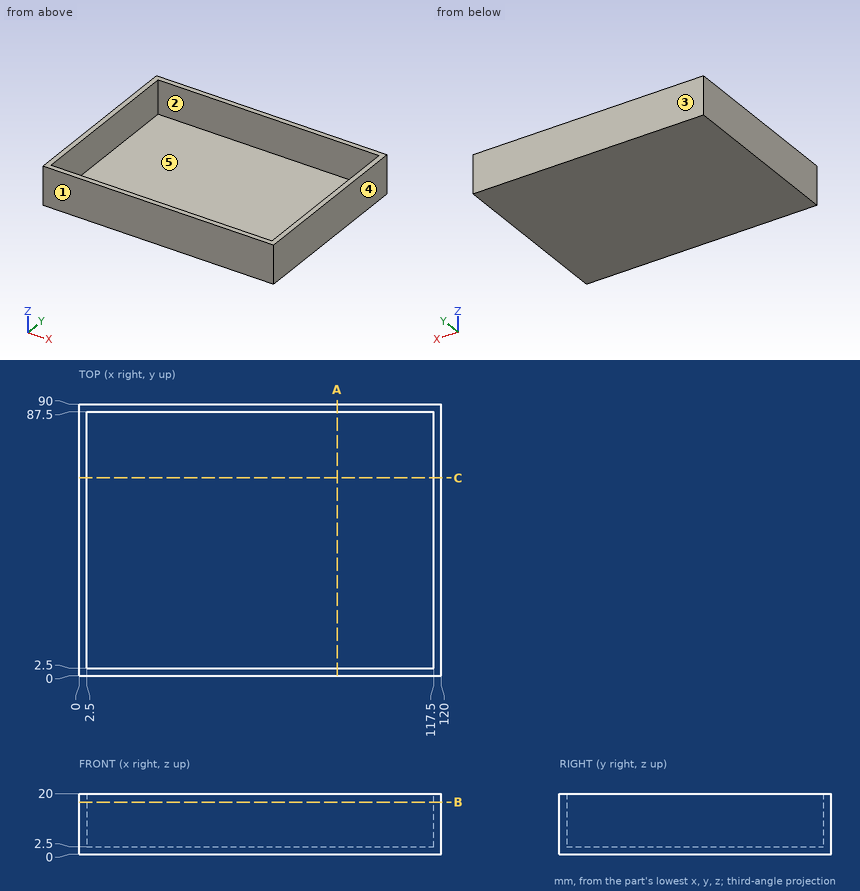
Answer from the drawing. Dimensions are ordinates in mm from the lowest x, y and z of the part. A direction names the side the tool comes from. Give positions to 0.01 mm unless a question says otherwise; leave off trailing zeros. Loops run counter-clockwise (first coordinate to the right, second up) from the corner with the lowest first, then second, coordinate; pieces in that order, holes last. Notation, with made-up numbers: (-20.5, 48.25) -> (28.5, 48.25) arc R9 cw to (28.5, 60.25) -> close; hole circle Ø6 at (-11, 76). An arc over 180 degrees is marked (long way). Use a Markdown table: item, result.
Q1. Section B-B, the plane z = 17.25 is taken. Determine the outline of the cut face in (x, y), then the cut area to 4 significant figures.
Solved:
| item | result |
|---|---|
| outline | (0, 0) -> (120, 0) -> (120, 90) -> (0, 90) -> close; hole (2.5, 2.5) -> (117.5, 2.5) -> (117.5, 87.5) -> (2.5, 87.5) -> close |
| area | 1,025 mm^2 |
Q2. Determine the mould class of the marked faces 1, 2 and 3 for opening direction Y: pulls with the +Y half, pulls with the -Y half, needs draft (parallel to the pull), parting line crosses it, or undercut.
Solved:
| item | result |
|---|---|
| face 1 | pulls with the -Y half |
| face 2 | undercut |
| face 3 | pulls with the +Y half |
Q3. Each of these flat-tipped pins is pushed along its axis until it touches: pin 1 (1 mm diameter, centred on x = 86, y = 74, fed in from -Z); pin 2 (6 mm diameter, centred on x = 15, y = 46, fed in from +Z). Where does it stop, or does it pass through?
Solved:
| item | result |
|---|---|
| pin 1 | stops at z = 0 |
| pin 2 | stops at z = 2.5 |
Q4. Find the intervals of material crossed by line 1 along Y through (x, z) = (50, 12.5); line 2 along X through (y, z) = (43, 5); line 3 along Z through (x, y) = (101.5, 74.5), in increasing order.
Solved:
| item | result |
|---|---|
| line 1 | y = 0 to 2.5, 87.5 to 90 |
| line 2 | x = 0 to 2.5, 117.5 to 120 |
| line 3 | z = 0 to 2.5 |
Q5. A tool of negligible diameter and unlimited length cuts with its end or side. For the marked faces 4 and 5, from which of +Z, -Z, +X, -X, +Y, -Y can it reach the whole face along a straight path? Write none if from no direction.
Solved:
| item | result |
|---|---|
| face 4 | +Z, -Z, +X, +Y, -Y |
| face 5 | +Z |
Q6. Section A-A, the plane x = 85.5 is taken. Determine the outline of the cut face in (y, z).
Solved:
| item | result |
|---|---|
| outline | (0, 0) -> (90, 0) -> (90, 20) -> (87.5, 20) -> (87.5, 2.5) -> (2.5, 2.5) -> (2.5, 20) -> (0, 20) -> close |
Q7. Section C-C, the plane y = 65.5 is taken. Determine the outline of the cut face in (x, z), then the cut area to 4 significant figures.
Solved:
| item | result |
|---|---|
| outline | (0, 0) -> (120, 0) -> (120, 20) -> (117.5, 20) -> (117.5, 2.5) -> (2.5, 2.5) -> (2.5, 20) -> (0, 20) -> close |
| area | 387.5 mm^2 |
